from build123d import *

# Parameters (mm, degrees)
SKETCH1_W               = 240
SKETCH1_H               = 175
BOSS_EXTRUDE1_DEPTH     = 40
CUT_EXTRUDE1_DEPTH      = 173.622771337
CUT_EXTRUDE1_DEPTH_BACK = 40
SKETCH3_W               = 5
SKETCH3_H               = 4.9
BOSS_EXTRUDE2_DEPTH     = 175
SHELL1_START            = 8.5
SHELL1_DEPTH            = 31.5
SKETCH4_R               = 2.65
SKETCH4_R_2             = 2.15
CUT_EXTRUDE2_DEPTH      = 8.5
CUT_EXTRUDE3_START      = -31.5
SKETCH5_W               = 5
SKETCH5_H               = 101.936090041
CUT_EXTRUDE3_DEPTH      = 31.5
SKETCH6_W               = 150
SKETCH6_H               = 2.9
SKETCH6_W_2             = 120
BOSS_EXTRUDE3_DEPTH     = 5
CUT_EXTRUDE4_REACH      = 277.406
SKETCH8_W               = 15
SKETCH8_H               = 25
BOSS_EXTRUDE4_DEPTH     = 10
CUT_EXTRUDE5_START      = -50
CUT_EXTRUDE5_DEPTH      = 50
BOSS_EXTRUDE5_DEPTH     = 31.5


# Read off the part's stored shape, not the designer's step: Shell1
with BuildPart() as part:
    # Sketch1 → Boss-Extrude1 (new body)
    with BuildSketch(Plane(origin=(0, 0, 0), x_dir=(1, 0, 0), z_dir=(0, 1, 0))):
        with Locations((0, 29.967532468)):
            Rectangle(SKETCH1_W, SKETCH1_H)
    extrude(amount=BOSS_EXTRUDE1_DEPTH)

    # Sketch2 → Cut-Extrude1 (cut, two sides: drawn at the far end of the back side and taken through both)
    with BuildSketch(Plane(origin=(0, 40, 0), x_dir=(1, 0, 0), z_dir=(0, 1, 0)).offset(-CUT_EXTRUDE1_DEPTH_BACK)):
        with BuildLine():
            Line((724.053869611, -57.532467532), (120, -57.532467532))
            Line((120, -57.532467532), (-82.377784234, -57.532467532))
            Line((-82.377784234, -57.532467532), (-120, 45.833720754))
            Line((-120, 45.833720754), (-30, 53.707700471))
            Line((-30, 53.707700471), (-19.393398282, 43.101098754))
            Line((-19.393398282, 43.101098754), (-39.130306901, 14.196870029))
            ThreePointArc((-39.130306901, 14.196870029), (-39.568663615, 6.465392529), (-32.936543603, 2.467532468))
            Line((-32.936543603, 2.467532468), (89.18584287, 2.467532468))
            Line((89.18584287, 2.467532468), (120, 117.467532468))
            Line((120, 117.467532468), (276.340645723, 700.938765595))
            Line((276.340645723, 700.938765595), (-764.036200619, 86.821246577))
            Line((-764.036200619, 86.821246577), (-316.322976731, -671.64998655))
            Line((-316.322976731, -671.64998655), (724.053869611, -57.532467532))
        make_face()
    extrude(amount=CUT_EXTRUDE1_DEPTH + CUT_EXTRUDE1_DEPTH_BACK, mode=Mode.SUBTRACT)

    # Sketch3 → Boss-Extrude2 (add)
    with BuildSketch(Plane.XY.offset(57.532467532)):
        with Locations((122.5, 20)):
            Rectangle(SKETCH3_W, SKETCH3_H)
    extrude(amount=-BOSS_EXTRUDE2_DEPTH)

    # Shell1 outline → Shell1 (cut)
    with BuildSketch(Plane(origin=(0, 0, 0), x_dir=(1, 0, 0), z_dir=(0, 1, 0)).offset(SHELL1_START)):
        with BuildLine():
            Line((111.5, -49.032467532), (111.5, 52.903622509))
            Line((111.5, 52.903622509), (95.708122268, -6.032467532))
            Line((95.708122268, -6.032467532), (-32.936543603, -6.032467532))
            ThreePointArc((-32.936543603, -6.032467532), (-47.085066295, 2.4963006), (-46.149905305, 18.990119265))
            Line((-46.149905305, 18.990119265), (-30.387255785, 42.074140976))
            Line((-30.387255785, 42.074140976), (-33.207708529, 44.89459372))
            Line((-33.207708529, 44.89459372), (-108.223913428, 38.331526211))
            Line((-108.223913428, 38.331526211), (-76.426020159, -49.032467532))
            Line((-76.426020159, -49.032467532), (111.5, -49.032467532))
        make_face()
    extrude(amount=SHELL1_DEPTH, mode=Mode.SUBTRACT)

    # Sketch4 → Cut-Extrude2 (cut)
    with BuildSketch(Plane(origin=(120, 0, 0), x_dir=(0, 0, -1), z_dir=(1, 0, 0))):
        with Locations((29.967532468, 30)):
            Circle(SKETCH4_R)
        with Locations((59.967532468, 30)):
            Circle(SKETCH4_R_2)
        with Locations((-20.032467532, 30)):
            Circle(SKETCH4_R_2)
        with Locations((29.967532468, 13.5)):
            Circle(SKETCH4_R)
        with Locations((59.967532468, 13.5)):
            Circle(SKETCH4_R_2)
        with Locations((-20.032467532, 13.5)):
            Circle(SKETCH4_R_2)
    extrude(amount=-CUT_EXTRUDE2_DEPTH, mode=Mode.SUBTRACT)

    # Sketch5 → Cut-Extrude3 (cut)
    with BuildSketch(Plane(origin=(0, 40, 0), x_dir=(1, 0, 0), z_dir=(0, 1, 0)).offset(CUT_EXTRUDE3_START)):
        with Locations((114, 1.935577488)):
            Rectangle(SKETCH5_W, SKETCH5_H)
    extrude(amount=CUT_EXTRUDE3_DEPTH, mode=Mode.SUBTRACT)

    # Sketch6 → Boss-Extrude3 (add)
    with BuildSketch(Plane(origin=(0, 40, 0), x_dir=(1, 0, 0), z_dir=(0, 1, 0))):
        with Locations((45, -53.282467532)):
            Rectangle(SKETCH6_W, SKETCH6_H)
        with Locations((30, -1.782467532)):
            Rectangle(SKETCH6_W_2, SKETCH6_H)
    extrude(amount=BOSS_EXTRUDE3_DEPTH)

    # Cut-Extrude4: up to this face of the body (flat: up to its plane)
    cut_extrude4_end = Plane(part.part.faces().sort_by_distance((116.5, 24.308295021, -1.744734026))[0])
    # Sketch8 → Cut-Extrude4 (cut, up to the picked face)
    with BuildSketch(Plane(origin=(125, 0, 0), x_dir=(0, 0, -1), z_dir=(1, 0, 0)), mode=Mode.PRIVATE) as cut_extrude4_sk1:
        with Locations((-32.532467532, 20)):
            Rectangle(SKETCH8_W, SKETCH8_H)
    cut_extrude4_tool1 = split(extrude(cut_extrude4_sk1.sketch, amount=-CUT_EXTRUDE4_REACH, mode=Mode.PRIVATE), bisect_by=cut_extrude4_end, keep=Keep.BOTH, mode=Mode.PRIVATE)
    add(cut_extrude4_tool1.solids().sort_by(Axis((125, 20, 32.532468), (-1, 0, 0)))[0], mode=Mode.SUBTRACT)


with BuildPart() as body_2:
    # Sketch9 → Boss-Extrude4 (new body)
    with BuildSketch(Plane(origin=(0, 40, 0), x_dir=(1, 0, 0), z_dir=(0, 1, 0))):
        with BuildLine():
            Line((120, -57.532467532), (120, 117.467532468))
            Line((120, 117.467532468), (89.18584287, 2.467532468))
            Line((89.18584287, 2.467532468), (-32.936543603, 2.467532468))
            ThreePointArc((-32.936543603, 2.467532468), (-39.568663615, 6.465392529), (-39.130306901, 14.196870029))
            Line((-39.130306901, 14.196870029), (-19.393398282, 43.101098754))
            Line((-19.393398282, 43.101098754), (-30, 53.707700471))
            Line((-30, 53.707700471), (-120, 45.833720754))
            Line((-120, 45.833720754), (-82.377784234, -57.532467532))
            Line((-82.377784234, -57.532467532), (120, -57.532467532))
        make_face()
    extrude(amount=BOSS_EXTRUDE4_DEPTH)


with BuildPart() as cut_extrude5_tool:
    # Sketch10 → Cut-Extrude5 (new body)
    with BuildSketch(Plane(origin=(0, 50, 0), x_dir=(1, 0, 0), z_dir=(0, 1, 0)).offset(CUT_EXTRUDE5_START)):
        Polygon((-120, 45.833720754), (-112.780643506, 46.465332605), (-74.928539827, -57.532467532), (-82.377784234, -57.532467532), align=None)
    extrude(amount=CUT_EXTRUDE5_DEPTH)


with BuildPart() as part_1:
    add(part.part)

    # Cut-Extrude5: cut by cut_extrude5_tool
    add(cut_extrude5_tool.part, mode=Mode.SUBTRACT)

    # Sketch11 → Boss-Extrude5 (add)
    with BuildSketch(Plane(origin=(0, 40, 0), x_dir=(1, 0, 0), z_dir=(0, 1, 0))):
        Polygon((-108.223913428, 38.331526211), (-100.488888614, 39.008253194), (-68.444686866, -49.032467532), (-76.426020159, -49.032467532), align=None)
    extrude(amount=-BOSS_EXTRUDE5_DEPTH)


with BuildPart() as body_2_1:
    add(body_2.part)

    # Cut-Extrude5: cut by cut_extrude5_tool
    add(cut_extrude5_tool.part, mode=Mode.SUBTRACT)


solid = part_1.part
Geometry: final body of the model. Coordinates: model frame, mm. A direction names the side the tool comes from. Give positions to 0.01 mm unless a question says otherwise; leave off trailing zeros. Loops run counter-clockwise (first coordinate to the right, second up) from the corner with the lowest first, then second, coordinate; pieces in that order, holes last. Notation, with made-up numbers: M 76,-30.75 L 82,-30.75 A13 cw 82,-14.75 Z; hole C 32.5,52 d7. An arc over 180 degrees is marked long. Put each result on its own line as item: value.
1) Cut plane B-B, the plane y = 3. Return the cut outline in (x, z), plus the area to 3 significant figures.
Computed values:
outline: M -112.78,-46.47 L -30,-53.71 L -19.39,-43.1 L -39.13,-14.2 A7.5 cw -32.94,-2.47 L 89.19,-2.47 L 120,-117.47 L 120,57.53 L -74.93,57.53 Z
area: 17,700 mm^2
2) Cut plane D-D, the plane z = -105.5. Return the cut outline in (x, y).
Computed values:
outline: M 116.79,0 L 120,0 L 120,17.55 L 125,17.55 L 125,22.45 L 120,22.45 L 120,40 L 116.79,40 Z
3) Mould query, pull axis Y, two halves, no side actions, for faces 1 (the flat face through (122, 20, -117.468)), 2 (the flat face through (122, 17.55, 49)), 3 (the flat face through (119, 20, 40.032)). Classes: released by +Y, released by -Y, zero draft, split by the parting line, or undercut.
Computed values:
face 1: zero draft
face 2: released by -Y
face 3: undercut
4) Reachability of faces 4 (the flat face through (-29.124, 19.72, -28.851)), 5 (the cylindrical face through (118.27, 11.15, -31.19)), 6 (the flat face through (29, 42, 3.232)), 7 (the flat face through (-38.38, 24.03, -30.37)), 8 (the flat face through (-24.77, 19.72, -48.48)) from +Z, -Z, +X, -X, +Y, -Y: full face, straight path, thin tool, end or side. Return the list, or none.
Computed values:
face 4: +Y, -Y
face 5: +X
face 6: +X, -X, +Y
face 7: +Y
face 8: -Z, +Y, -Y
5) Cut plane C-C, the plane z = -80. Return the cut outline in (x, y), plus the area to 3 significant figures.
Computed values:
outline: M 109.96,0 L 120,0 L 120,17.55 L 125,17.55 L 125,22.45 L 120,22.45 L 120,40 L 109.96,40 Z
area: 426 mm^2
6) Cut plane A-A, the plane x = 48. Return the cut outline in (y, z).
Computed values:
outline: M 0,-2.47 L 40,-2.47 L 40,0.33 L 45,0.33 L 45,3.23 L 40,3.23 L 40,6.03 L 8.5,6.03 L 8.5,49.03 L 40,49.03 L 40,51.83 L 45,51.83 L 45,54.73 L 40,54.73 L 40,57.53 L 0,57.53 Z
7) First-contact query: P1, Ø3.5, axis at y = 30, z = 20.03, coming from the -X side; P2, Ø4.5, axis at y = 29.5, z = -59.5, coming from the +X side; P3, Ø2.5, axis at x = 122, z = 47.5, coming from the -Y side. Flat tips, straight axial feed; report the tip coordinate or a pass-through.
Computed values:
P1: stops at x = -89.22
P2: stops at x = 120
P3: stops at y = 17.55
8) Material intervals for L1, parallel to Z at x = 30, y = 29; L2, parallel to X at y = 14, z = -12.5; L3, parallel to Z at x = -34, y = 22, sorted ascending. Write a range as from..to.
Computed values:
L1: z = -2.47..6.03, 49.03..57.53
L2: x = -100.42..-90.84, -48.73..-40, 91.87..100.67, 116.5..120
L3: z = -53.36..-44.83, -36.78..-21.71, -2.54..6, 49.03..57.53
